```python
from build123d import *

# Parameters (mm, degrees)
ESQUISSE1_W             = 70
ESQUISSE1_H             = 80
ESQUISSE1_R             = 3.3
ESQUISSE1_R_2           = 2.75
BOSS_EXTRU_1_DEPTH      = 10
ESQUISSE2_R             = 6
ENL_V_MAT_EXTRU_1_DEPTH = 5
ENL_V_MAT_EXTRU_3_DEPTH = 7


with BuildPart() as part:
    # Esquisse1 → Boss.-Extru.1 (new body)
    with BuildSketch(Plane.XY):
        with Locations((-26.178136106, 1.138047212)):
            Rectangle(ESQUISSE1_W, ESQUISSE1_H)
        with Locations((0.821863894, 24.138047212)):
            Circle(ESQUISSE1_R, mode=Mode.SUBTRACT)
        with Locations((-12.178136106, 24.138047212)):
            Circle(ESQUISSE1_R, mode=Mode.SUBTRACT)
        with Locations((-12.178136106, -21.861952788)):
            Circle(ESQUISSE1_R, mode=Mode.SUBTRACT)
        with Locations((0.821863894, -21.861952788)):
            Circle(ESQUISSE1_R, mode=Mode.SUBTRACT)
        with Locations((-51.178136106, 31.138047212)):
            Circle(ESQUISSE1_R_2, mode=Mode.SUBTRACT)
        with Locations((-31.178136106, 31.138047212)):
            Circle(ESQUISSE1_R_2, mode=Mode.SUBTRACT)
        with Locations((-31.178136106, -28.861952788)):
            Circle(ESQUISSE1_R_2, mode=Mode.SUBTRACT)
        with Locations((-51.178136106, -28.861952788)):
            Circle(ESQUISSE1_R_2, mode=Mode.SUBTRACT)
    extrude(amount=BOSS_EXTRU_1_DEPTH)

    # Esquisse2 → Enlèv. mat.-Extru.1 (cut)
    with BuildSketch(Plane.XY.offset(10)):
        with Locations((-51.178136106, 31.138047212)):
            Circle(ESQUISSE2_R)
        with Locations((-31.178136106, 31.138047212)):
            Circle(ESQUISSE2_R)
        with Locations((-31.178136106, -28.861952788)):
            Circle(ESQUISSE2_R)
        with Locations((-51.178136106, -28.861952788)):
            Circle(ESQUISSE2_R)
    extrude(amount=-ENL_V_MAT_EXTRU_1_DEPTH, mode=Mode.SUBTRACT)

    # Esquisse3 → Enlèv. mat.-Extru.3 (cut)
    with BuildSketch(Plane(origin=(0, 0, 0), x_dir=(-1, 0, 0), z_dir=(0, 0, -1))):
        with BuildLine():
            Line((-0.821863894, 31.138047212), (12.178136106, 31.138047212))
            ThreePointArc((12.178136106, 31.138047212), (19.178136106, 24.138047212), (12.178136106, 17.138047212))
            Line((12.178136106, 17.138047212), (-0.821863894, 17.138047212))
            ThreePointArc((-0.821863894, 17.138047212), (-7.821863894, 24.138047212), (-0.821863894, 31.138047212))
        make_face()
        with BuildLine():
            Line((-0.821863894, -14.861952788), (12.178136106, -14.861952788))
            ThreePointArc((12.178136106, -14.861952788), (19.178136106, -21.861952788), (12.178136106, -28.861952788))
            Line((12.178136106, -28.861952788), (-0.821863894, -28.861952788))
            ThreePointArc((-0.821863894, -28.861952788), (-7.821863894, -21.861952788), (-0.821863894, -14.861952788))
        make_face()
    extrude(amount=-ENL_V_MAT_EXTRU_3_DEPTH, mode=Mode.SUBTRACT)


solid = part.part
```
The listing builds one solid part. Answer for the finished solid, in the listing's coordinates (mm). A direction names the side the tool comes from. Give positions to 0.01 mm unless a question says otherwise; leave off trailing zeros. Order: outer loops, then holes, each group sorted by start corner. A loop starts at its lowest first (then second) coordinate and runs counter-clockwise, first axis right, second up. Notation, with made-up numbers: (41.25, -10) -> (55.25, -10) arc R9 ccw to (55.25, -4) -> close; hole circle Ø1 at (51, 70). An arc over 180 degrees is marked (long way). Answer as a JSON object with one key per item and string values. Group by question number.
Item 1: The part is cut by section D-D on z = 8.5. Give the number of separate pieces and of enclosed holes in the cut face, and give its area (3 significant figures).
Item 2: A tool of negligible diameter and unlimited length cuts with its end or side. For faces 1 (the flat face through (8.822, 1, 5)), 2 (the cylindrical face through (-45.636, 28.84, 7.535)), 3 (the cylindrical face through (7.82, -22.02, 3.45)), from which of +Z, -Z, +X, -X, +Y, -Y can it reach the whole face along a straight path? Write none if from no direction.
Item 3: Flat-ended cylindrical pins translate along their axes: pin 1 (1.5 mm diameter, centred on x = -14.5, y = 29.5, fed in from -Z); pin 2 (6.5 mm diameter, centred on x = -51.18, y = -28.86, fed in from +Z). Find the tip coordinate at first contact, or state that the pin passes through.
Item 4: The part is cut by section A-A on z = 3.5. Write down the section's boundary in (x, y), and give its area (3 significant figures).
Item 5: Consider L1, parallel to Y at x = -32, z = 1.75; L2, parallel to Y at x = -51, z = 3; L3, parallel to X at y = 30, z = 9.5. Determine where each line is inside the solid, lowest interval first. Write a range as from..to.
Item 6: The part is cut by section B-B on y = 29.5. Write down the section's boundary in (x, z).
Item 7: Determine the mould class of faces 4 (the flat face through (-61.178, 1, 5)), 5 (the flat face through (-6, 17.138, 3)), 6 (the cylindrical face through (3.87, 22.87, 8.48)), 7 (the flat face through (-34, 2, 0)) for opening direction X: pulls with the +X half, pulls with the -X half, needs draft (parallel to the pull), parting line crosses it, or undercut.
Item 8: The part is cut by section C-C on x = -55. Write down the section's boundary in (y, z).
Result set:
{
 "1": {"separate pieces": "1", "enclosed holes": "8", "area": "5,010 mm²"},
 "2": {"face 1": "+Z, -Z, +X, +Y, -Y", "face 2": "+Z", "face 3": "-Z"},
 "3": {"pin 1": "z = 7", "pin 2": "z = 5"},
 "4": {"outline": "(-61.18, -38.86) -> (8.82, -38.86) -> (8.82, 41.14) -> (-61.18, 41.14) -> close; hole circle Ø5.5 at (-51.18, -28.86); hole circle Ø5.5 at (-51.18, 31.14); hole circle Ø5.5 at (-31.18, -28.86); hole circle Ø5.5 at (-31.18, 31.14); hole (-12.18, -28.86) -> (0.82, -28.86) arc R7 ccw to (0.82, -14.86) -> (-12.18, -14.86) arc R7 ccw to start; hole (-12.18, 17.14) -> (0.82, 17.14) arc R7 ccw to (0.82, 31.14) -> (-12.18, 31.14) arc R7 ccw to start", "area": "4,830 mm²"},
 "5": {"L1": "-38.86..-31.49, -26.24..28.51, 33.76..41.14", "L2": "-38.86..-31.61, -26.12..28.39, 33.88..41.14", "L3": "-61.18..-57.07, -45.29..-37.07, -25.29..8.82"},
 "6": {"outline": "(-61.18, 0) -> (-53.39, 0) -> (-53.39, 5) -> (-56.95, 5) -> (-56.95, 10) -> (-61.18, 10) -> close; (-48.97, 0) -> (-33.39, 0) -> (-33.39, 5) -> (-36.95, 5) -> (-36.95, 10) -> (-45.41, 10) -> (-45.41, 5) -> (-48.97, 5) -> close; (-28.97, 0) -> (-16.68, 0) -> (-16.68, 7) -> (5.32, 7) -> (5.32, 0) -> (8.82, 0) -> (8.82, 10) -> (-25.41, 10) -> (-25.41, 5) -> (-28.97, 5) -> close"},
 "7": {"face 4": "pulls with the -X half", "face 5": "undercut", "face 6": "undercut", "face 7": "needs draft"},
 "8": {"outline": "(-38.86, 0) -> (41.14, 0) -> (41.14, 10) -> (35.76, 10) -> (35.76, 5) -> (26.51, 5) -> (26.51, 10) -> (-24.24, 10) -> (-24.24, 5) -> (-33.49, 5) -> (-33.49, 10) -> (-38.86, 10) -> close"}
}
